Read the model definition and answer for the solid it produces. Units are mm, in the model's axes. Face numbers are marked on the shaded views. A direction names the side the tool comes from. Round coordinates to 2 decimals unless told otherwise and drop trailing zeros. Loops run counter-clockwise (first coordinate to the right, second up) from the corner with the lowest first, then second, coordinate; pieces in that order, holes last. Notation, with made-up numbers: (-7.5, -37.5) -> (32.5, -37.5) arc R16 ccw to (32.5, -15.5) -> close; hole circle Ø8 at (-9, 53). An arc over 180 degrees is marked (long way). Put each result on its own line as item: value.
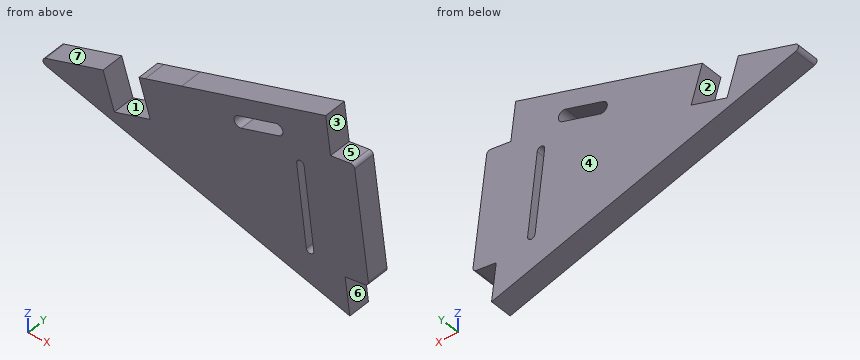
from build123d import *

# Parameters (mm, degrees)
BOSS_EXTRUDE1_DEPTH = 6
FILLET1_R           = 1
CUT_EXTRUDE1_DEPTH  = 93.288252623


with BuildPart() as part:
    # Sketch1 → Boss-Extrude1 (new body)
    with BuildSketch(Plane(origin=(0, 0, 0), x_dir=(1, 0, 0), z_dir=(0, 1, 0))):
        Polygon((-2.58662904, -0.182978259), (-1.306630871, 9.734763655), (4.991135245, 8.921964817), (8.862776708, 38.921964817), (2.565209371, 39.734738), (3.813361808, 49.405731314), (-80.122978657, 24.047130996), (-50.562245366, 14.809401842), (-40.870201664, 11.780638185), align=None)
        with BuildLine():
            Line((-5.765677194, 37.231163577), (-8.327046549, 16.028717249))
            ThreePointArc((-8.327046549, 16.028717249), (-9.439761879, 15.155868697), (-10.312610431, 16.268584027))
            Line((-10.312610431, 16.268584027), (-7.751241076, 37.471030354))
            ThreePointArc((-7.751241076, 37.471030354), (-6.638525747, 38.343878906), (-5.765677194, 37.231163577))
        make_face(mode=Mode.SUBTRACT)
    extrude(amount=BOSS_EXTRUDE1_DEPTH)

    # Fillet1
    fillet1_edges = [part.edges().sort_by_distance(p)[0] for p in [
        (-80.122978657, 3, -24.047130996),
        (8.862776708, 3, -38.921964817),
        (4.991135245, 3, -8.921964817),
    ]]
    fillet(fillet1_edges, radius=FILLET1_R)

    # Sketch2 → Cut-Extrude1 (cut, through all)
    with BuildSketch(Plane(origin=(0, 6, 0), x_dir=(1, 0, 0), z_dir=(0, 1, 0))):
        Polygon((-61.745288627, 18.304102861), (-58.762538695, 27.848902642), (-49.217738915, 24.86615271), (-52.200488846, 15.32135293), align=None)
        with BuildLine():
            Line((-25.001158575, 14.705103686), (-15.001158575, 11.580103686))
            ThreePointArc((-15.001158575, 11.580103686), (-14.016851097, 9.70097123), (-15.895983554, 8.716663752))
            Line((-15.895983554, 8.716663752), (-25.895983554, 11.841663752))
            ThreePointArc((-25.895983554, 11.841663752), (-26.880291031, 13.720796209), (-25.001158575, 14.705103686))
        make_face()
    extrude(amount=-CUT_EXTRUDE1_DEPTH, mode=Mode.SUBTRACT)


solid = part.part
Item 1: The part is cut by section A-A (y = 4.05). Determine the outline of the cut face in (x, z).
Derived:
outline: (-77.02, -23.08) arc R1 ccw to (-77.01, -24.99) -> (3.81, -49.41) -> (2.57, -39.73) -> (7.87, -39.05) arc R1 ccw to (8.73, -37.93) -> (5.12, -9.91) arc R1 ccw to (4, -9.05) -> (-1.31, -9.73) -> (-2.59, 0.18) -> (-52.2, -15.32) -> (-49.22, -24.87) -> (-58.76, -27.85) -> (-61.75, -18.3) -> close; hole (-25.9, -11.84) arc R1.5 ccw to (-25, -14.71) -> (-15, -11.58) arc R1.5 ccw to (-15.9, -8.72) -> close; hole (-10.31, -16.27) -> (-7.75, -37.47) arc R1 ccw to (-5.77, -37.23) -> (-8.33, -16.03) arc R1 ccw to start
Item 2: For a pull along Z with two mould halves and no side action, classify the marked faces 1, 2, 3 and 4 as pulls with the +Z half, pulls with the -Z half, needs draft (parallel to the pull), parting line crosses it, or undercut.
Derived:
face 1: undercut
face 2: undercut
face 3: pulls with the +Z half
face 4: needs draft
Item 3: Find the intervals of material crossed by line 1 along X through (y, z) = (2.8, -17); line 2 along Z through (x, y) = (-20.5, 3.7); line 3 along Z through (x, y) = (-32, 4.95), in increasing order.
Derived:
line 1: x = -51.68 to -10.22, -8.21 to 6.03
line 2: z = -42.06 to -13.3, -10.16 to -5.41
line 3: z = -38.59 to -9.01
Item 4: The part is cut by section C-C (x = -47.5). Determine the outline of the cut face in (y, z).
Derived:
outline: (0, -33.9) -> (6, -33.9) -> (6, -13.85) -> (0, -13.85) -> close
Item 5: Flat-ended cylindrical pins translate along their axes: pin 1 Ø2 at (x, y) = (-41.5, 2) entering from -Z; pin 2 Ø1 at (y, z) = (1.5, -19) entering from +X. Find the tip coordinate at first contact, or state that the pin passes through.
Derived:
pin 1: stops at z = -36.02
pin 2: stops at x = 6.36
Item 6: The part is cut by section B-B (z = -34.5). Determine the outline of the cut face in (x, y).
Derived:
outline: (-45.52, 0) -> (-8.11, 0) -> (-8.11, 6) -> (-45.52, 6) -> close; (-6.1, 0) -> (8.29, 0) -> (8.29, 6) -> (-6.1, 6) -> close
Item 7: Which of the six approach directions +Z, -Z, +X, -X, +Y, -Y give full straight-line access (tool end or side, diameter ignored) to the marked faces 5, 6 and 7?
Derived:
face 5: +Z, +Y, -Y
face 6: +X, +Y, -Y
face 7: +Z, -X, +Y, -Y
Item 8: The part is cut by section D-D (z = -7). Determine the outline of the cut face in (x, y).
Derived:
outline: (-25.57, 0) -> (-1.66, 0) -> (-1.66, 6) -> (-25.57, 6) -> close
